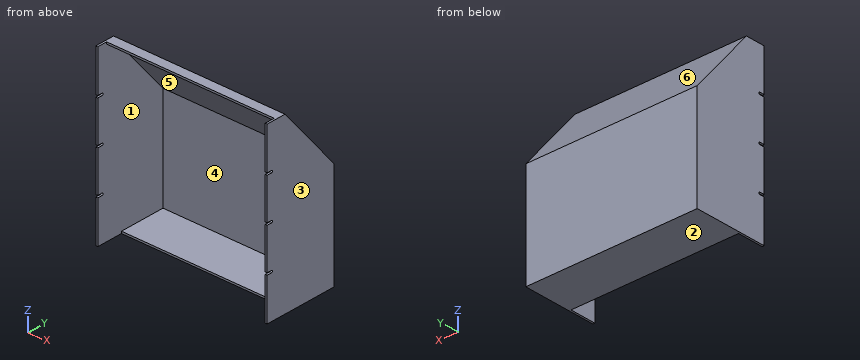
```python
from build123d import *

# Parameters (mm, degrees)
ESTRUSIONE_ESTRUSIONE1_DEPTH = 524
SVUOTA1_T                    = -6
SCHIZZO2_W                   = 512
SCHIZZO2_H                   = 6
TAGLIO_ESTRUSIONE1_DEPTH     = 30
SCHIZZO3_W                   = 512
SCHIZZO3_H                   = 6
TAGLIO_ESTRUSIONE2_DEPTH     = 80
TAGLIO_ESTRUSIONE3_DEPTH     = 775.74382863


with BuildPart() as part:
    # Schizzo1 → Estrusione-Estrusione1 (new body)
    with BuildSketch(Plane(origin=(0, 0, 0), x_dir=(0, 0, -1), z_dir=(1, 0, 0))):
        Polygon((524, 0), (524, 226), (201.576132106, 226), (0, 60), (0, 0), align=None)
    extrude(amount=ESTRUSIONE_ESTRUSIONE1_DEPTH)

    # Svuota1
    svuota1_openings = [part.faces().sort_by_distance(p)[0] for p in [
        (262, 0, -262),
    ]]
    offset(amount=SVUOTA1_T, openings=svuota1_openings, kind=Kind.INTERSECTION)

    # Schizzo2 → Taglio-Estrusione1 (cut)
    with BuildSketch(Plane.XZ):
        with Locations((262, -3)):
            Rectangle(SCHIZZO2_W, SCHIZZO2_H)
    extrude(amount=-TAGLIO_ESTRUSIONE1_DEPTH, mode=Mode.SUBTRACT)

    # Schizzo3 → Taglio-Estrusione2 (cut)
    with BuildSketch(Plane.XZ):
        with Locations((262, -521)):
            Rectangle(SCHIZZO3_W, SCHIZZO3_H)
    extrude(amount=-TAGLIO_ESTRUSIONE2_DEPTH, mode=Mode.SUBTRACT)

    # Schizzo4 → Taglio-Estrusione3 (cut, through all)
    with BuildSketch(Plane.ZY):
        with BuildLine():
            Line((-396.25, 15), (-396.25, 0))
            Line((-396.25, 0), (-389.75, 0))
            Line((-389.75, 0), (-389.75, 15))
            ThreePointArc((-389.75, 15), (-393, 18.25), (-396.25, 15))
        make_face()
        with BuildLine():
            Line((-265.25, 15), (-265.25, 0))
            Line((-265.25, 0), (-258.75, 0))
            Line((-258.75, 0), (-258.75, 15))
            ThreePointArc((-258.75, 15), (-262, 18.25), (-265.25, 15))
        make_face()
        with BuildLine():
            Line((-134.25, 0), (-127.75, 0))
            Line((-127.75, 0), (-127.75, 15))
            ThreePointArc((-127.75, 15), (-131, 18.25), (-134.25, 15))
            Line((-134.25, 15), (-134.25, 0))
        make_face()
    extrude(amount=-TAGLIO_ESTRUSIONE3_DEPTH, mode=Mode.SUBTRACT)


solid = part.part
```
Read the model definition and answer for the solid it produces. Units are mm, in the model's axes. Face numbers are marked on the shaded views. A direction names the side the tool comes from. Coordinates: 2 decimals unless noted, no trailing zeros. Loops run counter-clockwise (first coordinate to the right, second up) from the corner with the lowest first, then second, coordinate; pieces in that order, holes last.
(1) Flat-ended cylindrical pins translate along their axes: pin 1 Ø1.5 at (y, z) = (109.5, -418.5) entering from -X; pin 2 Ø1.5 at (x, z) = (426.5, -130) entering from +Y; pin 3 Ø10 at (x, z) = (327.5, -201.5) entering from -Y; pin 4 Ø6.5 at (x, z) = (200.5, -2.5) entering from -Y. Find the tip coordinate at first contact, or state that the pin passes through.
Solution:
pin 1: stops at x = 0
pin 2: stops at y = 167.67
pin 3: stops at y = 214.05
pin 4: stops at y = 30
(2) The mould has two halves that part along X. Classify the marked faces 3, 4, 5 and 6: released by +X, released by -X, zero draft, split by the parting line, or undercut.
Solution:
face 3: released by +X
face 4: undercut
face 5: undercut
face 6: zero draft
(3) The part is cut by section D-D (y = 40). Determine the outline of the cut face in (x, z), and give its area (3 significant figures).
Solution:
outline: (0, -524) - (6, -524) - (6, -6) - (518, -6) - (518, -524) - (524, -524) - (524, 0) - (0, 0) - close
area: 9,360 mm2
(4) Consider line 1 along X through (y, z) = (142, -184); line 2 along Z through (x, y) = (408.5, 36.5); line 3 along Y through (x, z) = (449, -377). Determine where each line is inside the solid, lowest interval first.
Solution:
line 1: x = 0 to 6, 518 to 524
line 2: z = -6 to 0
line 3: y = 220 to 226
(5) A tool of negligible diameter and unlimited length cuts with its end or side. For the marked faces 1 and 2, from which of +Z, -Z, +X, -X, +Y, -Y can it reach the whole face along a straight path? Write none if from no direction.
Solution:
face 1: -Y
face 2: -Z, +X, -X, +Y, -Y
(6) The part is cut by section A-A (y = 140). Determine the outline of the cut face in (x, z).
Solution:
outline: (0, -524) - (524, -524) - (524, -97.15) - (0, -97.15) - close; hole (6, -518) - (518, -518) - (518, -106.58) - (6, -106.58) - close
(7) The part is cut by section C-C (z = -278.5). Determine the outline of the cut face in (x, y).
Solution:
outline: (0, 0) - (6, 0) - (6, 220) - (518, 220) - (518, 0) - (524, 0) - (524, 226) - (0, 226) - close
(8) The part is cut by section B-B (x = 362). Determine the outline of the cut face in (y, z), and give its area (3 significant figures).
Solution:
outline: (30, -6) - (57.17, -6) - (220, -203.73) - (220, -518) - (80, -518) - (80, -524) - (226, -524) - (226, -201.58) - (60, 0) - (30, 0) - close
area: 4,490 mm2
